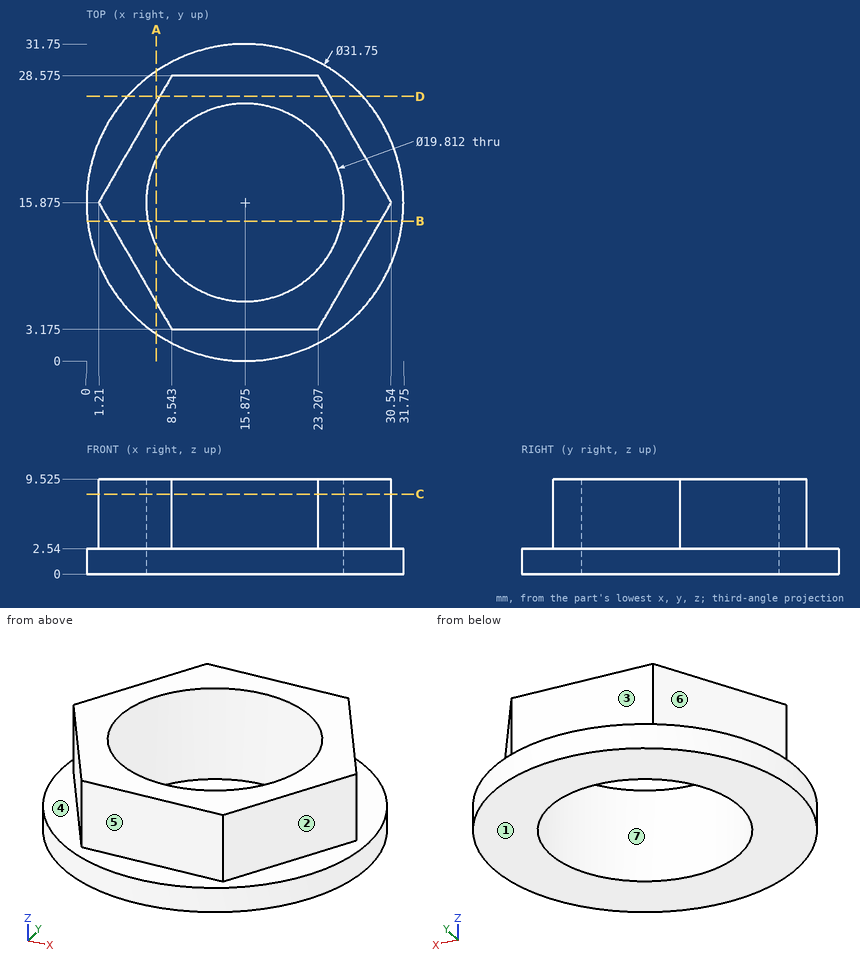
Check sheet for the drawn part. Datum: minimum x, y, z corner. Units: mm. A direction names the side the tool comes from. Coordinates: 2 decimals unless noted, no trailing zeros. Order: outer loops, then holes, each group sorted by start corner. A loop starts at its lowest first (then second) coordinate and runs counter-clockwise, first axis right, second up. Notation, with made-up numbers: (19.25, 7.5) - (70.25, 7.5) arc R8 cw to (70.25, 21.5) - close; hole circle Ø8 at (-31, 76). An arc over 180 degrees is marked (long way). Return JSON: item names as keys, results as strings.
(1) Section check C-C, the plane z = 8. Record the cut outline in (x, y) (1 decimal).
Filled sheet:
{"outline": "(1.2, 15.9) - (8.5, 3.2) - (23.2, 3.2) - (30.5, 15.9) - (23.2, 28.6) - (8.5, 28.6) - close; hole circle Ø19.8 at (15.9, 15.9)"}
(2) Thickness scan on line 1 along X through (y, z) = (15, 8.5) (1 decimal); line 2 along Y through (x, z) = (13, 2.75) (1 decimal); line 3 along Z through (x, y) = (4, 10.5). Record the ranges inside material, lowest first.
Filled sheet:
{"line 1": "x = 1.7 to 6, 25.7 to 30", "line 2": "y = 3.2 to 6.4, 25.4 to 28.6", "line 3": "z = 0 to 2.54"}
(3) Access from +Z, -Z, +X, -X, +Y, -Y to the whole of each face (thin tool, end or side, straight path). Record for the marked faces 1, 2 and 3.
Filled sheet:
{"face 1": "-Z, +X, -X, +Y, -Y", "face 2": "+Z, +X, -Y", "face 3": "+Z, +X, -X, +Y"}
(4) Mould release check, pull along Y, two halves, no side actions. Record for the marked faces 4, 5, 6 and 7: pulls with the +Y half, pulls with the -Y half, needs draft (parallel to the pull), parting line crosses it, or undercut.
Filled sheet:
{"face 4": "needs draft", "face 5": "pulls with the -Y half", "face 6": "pulls with the +Y half", "face 7": "undercut"}
(5) Go/stop test with flat-tipped pins: pin 1 (2 mm diameter, centred on x = 5.5, z = 2, fed in from +Y) (1 decimal); pin 2 (16 mm diameter, centred on x = 15.875, y = 15.875, fed in from -Z); pin 3 (4 mm diameter, centred on x = 20.5, z = 6, fed in from +Y) (3 decimals); pin 4 (5 mm diameter, centred on x = 15.5, z = 1.5, fed in from +Y). Record where each tip stops, or that it passes through.
Filled sheet:
{"pin 1": "stops at y = 28.7", "pin 2": "passes through", "pin 3": "stops at y = 28.575", "pin 4": "stops at y = 31.75"}
(6) Section check B-B, the plane y = 14. Record the cut outline in (x, z) (1 decimal).
Filled sheet:
{"outline": "(0.1, 0) - (6.1, 0) - (6.1, 9.5) - (2.3, 9.5) - (2.3, 2.5) - (0.1, 2.5) - close; (25.6, 0) - (31.6, 0) - (31.6, 2.5) - (29.5, 2.5) - (29.5, 9.5) - (25.6, 9.5) - close"}
(7) Section check D-D, the plane y = 26.5. Record the cut outline in (x, z) (1 decimal), and give its area (3 significant figures).
Filled sheet:
{"outline": "(4.1, 0) - (27.7, 0) - (27.7, 2.5) - (24.4, 2.5) - (24.4, 9.5) - (7.3, 9.5) - (7.3, 2.5) - (4.1, 2.5) - close", "area": "179 mm^2"}
(8) Section check A-A, the plane x = 7. Record the cut outline in (y, z) (1 decimal), and give its area (3 significant figures).
Filled sheet:
{"outline": "(2.7, 0) - (11.5, 0) - (11.5, 9.5) - (5.8, 9.5) - (5.8, 2.5) - (2.7, 2.5) - close; (20.3, 0) - (29, 0) - (29, 2.5) - (25.9, 2.5) - (25.9, 9.5) - (20.3, 9.5) - close", "area": "123 mm^2"}
